```python
from build123d import *

# Parameters (mm, degrees)
ESTRUSIONE_SOTTILE1_DEPTH    = 210
SCHIZZO2_W                   = 20
SCHIZZO2_H                   = 30
SCHIZZO2_R                   = 4.25
ESTRUSIONE_ESTRUSIONE1_DEPTH = 1.5


with BuildPart() as part:
    # Schizzo1 → Estrusione-Sottile1 (new body)
    with BuildSketch(Plane(origin=(0, 0, 0), x_dir=(1, 0, 0), z_dir=(0, 1, 0))):
        with BuildLine():
            Line((0, 125), (0, 10))
            ThreePointArc((0, 10), (2.928932188, 2.928932188), (10, 0))
            Line((10, 0), (254, 0))
            ThreePointArc((254, 0), (261.071067812, 2.928932188), (264, 10))
            Line((264, 10), (264, 125))
            ThreePointArc((264, 125), (261.071067812, 132.071067812), (254, 135))
            Line((254, 135), (10, 135))
            ThreePointArc((10, 135), (2.928932188, 132.071067812), (0, 125))
        make_face()
        with BuildLine():
            Line((1.5, 125), (1.5, 10))
            ThreePointArc((1.5, 10), (3.98959236, 3.98959236), (10, 1.5))
            Line((10, 1.5), (254, 1.5))
            ThreePointArc((254, 1.5), (260.01040764, 3.98959236), (262.5, 10))
            Line((262.5, 10), (262.5, 125))
            ThreePointArc((262.5, 125), (260.01040764, 131.01040764), (254, 133.5))
            Line((254, 133.5), (10, 133.5))
            ThreePointArc((10, 133.5), (3.98959236, 131.01040764), (1.5, 125))
        make_face(mode=Mode.SUBTRACT)
    extrude(amount=ESTRUSIONE_SOTTILE1_DEPTH)

    # Schizzo2 → Estrusione-Estrusione1 (add)
    # profile 1 of 2: a face of its own
    with BuildSketch(Plane(origin=(0, 210, 0), x_dir=(1, 0, 0), z_dir=(0, 1, 0))):
        with Locations((11.5, 67.5)):
            Rectangle(SCHIZZO2_W, SCHIZZO2_H)
        with Locations(Location((11.5, 67.5, 0), (0, 0, 270))):
            Circle(SCHIZZO2_R, mode=Mode.SUBTRACT)
    # profile 2 of 2: a face of its own
    with BuildSketch(Plane(origin=(0, 210, 0), x_dir=(1, 0, 0), z_dir=(0, 1, 0))):
        with Locations((252.5, 67.5)):
            Rectangle(SCHIZZO2_W, SCHIZZO2_H)
        with Locations(Location((252.5, 67.5, 0), (0, 0, 90))):
            Circle(SCHIZZO2_R, mode=Mode.SUBTRACT)
    extrude(amount=-ESTRUSIONE_ESTRUSIONE1_DEPTH)


solid = part.part
```
Source: CAD feature listing. Evaluate the final solid. Frame: model axes, mm. A direction names the side the tool comes from. Round coordinates to 2 decimals unless told otherwise and drop trailing zeros. Loops run counter-clockwise (first coordinate to the right, second up) from the corner with the lowest first, then second, coordinate; pieces in that order, holes last.
(1) Section query D-D (y = 165.5). Output: boundary loops of the cut face in (x, z).
From the geometry:
outline: (0, -125) arc R10 ccw to (10, -135) - (254, -135) arc R10 ccw to (264, -125) - (264, -10) arc R10 ccw to (254, 0) - (10, 0) arc R10 ccw to (0, -10) - close; hole (1.5, -125) arc R8.5 ccw to (10, -133.5) - (254, -133.5) arc R8.5 ccw to (262.5, -125) - (262.5, -10) arc R8.5 ccw to (254, -1.5) - (10, -1.5) arc R8.5 ccw to (1.5, -10) - close
(2) Material intervals for probe 1 along Z at (x, y) = (252.5, 209.2); probe 2 along X at (y, z) = (209, -67); probe 3 along X at (y, z) = (141.5, -63), sorted ascending.
From the geometry:
probe 1: z = -135 to -133.5, -82.5 to -71.75, -63.25 to -52.5, -1.5 to 0
probe 2: x = 0 to 7.28, 15.72 to 21.5, 242.5 to 248.28, 256.72 to 264
probe 3: x = 0 to 1.5, 262.5 to 264
(3) Pull-direction query (X, two-part tool) for faces 4 (the flat face through (14, 210, -73)), 5 (the cylindrical face through (3.92, 103.53, -4.06)), 6 (the cylindrical face through (3.01, 103.53, -132.15)), 7 (the cylindrical face through (4.06, 103.53, -131.08)); classes: +X half, -X half, draft (parallel to the pull), parting line (faces both ways), or undercut.
From the geometry:
face 4: draft
face 5: undercut
face 6: -X half
face 7: undercut
(4) Section query B-B (z = -97.5). Output: boundary loops of the cut face in (x, y).
From the geometry:
outline: (0, 0) - (1.5, 0) - (1.5, 210) - (0, 210) - close; (262.5, 0) - (264, 0) - (264, 210) - (262.5, 210) - close
(5) Section query C-C (x = 115.5). Output: boundary loops of the cut face in (y, z), and give its area (3 significant figures).
From the geometry:
outline: (0, -135) - (210, -135) - (210, -133.5) - (0, -133.5) - close; (0, -1.5) - (210, -1.5) - (210, 0) - (0, 0) - close
area: 630 mm2
(6) Access query for faces 1 (the flat face through (262.5, 104, -67)), 2 (the cylindrical face through (260.08, 103.53, -130.94)), 3 (the cylindrical face through (2.85, 103.53, -3.01)). Directions: +Z, -Z, +X, -X, +Y, -Y. A direction counts if a zero-diameter tool reaches every point of the face in a straight line with its end or side. Return the directions, or none.
From the geometry:
face 1: -Y
face 2: +Y, -Y
face 3: +Z, -X, +Y, -Y
(7) Contact query for flat-ended pins moving along their axis: pin 1 Ø1.6 at (x, y) = (256, 209.5) entering from -Z; pin 2 Ø6 at (x, z) = (249.5, -60.5) entering from -Y; pin 3 Ø1.2 at (x, y) = (9.5, 209.5) entering from -Z. Output: stop coordinate, or through.
From the geometry:
pin 1: stops at z = -134.93
pin 2: stops at y = 208.5
pin 3: stops at z = -135
(8) Section query A-A (z = -67.5). Output: boundary loops of the cut face in (x, y), and give its area (4 significant figures).
From the geometry:
outline: (0, 0) - (1.5, 0) - (1.5, 208.5) - (7.25, 208.5) - (7.25, 210) - (0, 210) - close; (15.75, 208.5) - (21.5, 208.5) - (21.5, 210) - (15.75, 210) - close; (242.5, 208.5) - (248.25, 208.5) - (248.25, 210) - (242.5, 210) - close; (256.75, 208.5) - (262.5, 208.5) - (262.5, 0) - (264, 0) - (264, 210) - (256.75, 210) - close
area: 664.5 mm2
